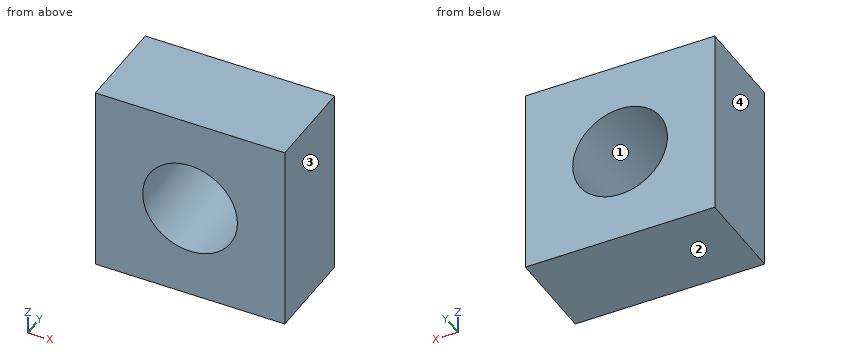
```python
from build123d import *

# Parameters (mm, degrees)
F0_W     = 20
F0_H     = 20
F1_DEPTH = 10
F2_R     = 5
F3_DEPTH = 10.001


with BuildPart() as f1:
    # F0 (on Front) → F1 (new body)
    with BuildSketch(Plane.XZ):
        Rectangle(F0_W, F0_H)
    extrude(amount=F1_DEPTH)

    # F2 (on face) → F3 (cut, through all)
    with BuildSketch(Plane.XZ.offset(10)):
        Circle(F2_R)
    extrude(amount=-F3_DEPTH, mode=Mode.SUBTRACT)


solid = f1.part
```
Geometry check sheet. Reference: the model listing, model coordinates, mm. Face numbers are marked on the shaded views. Give positions to 0.01 mm unless a question says otherwise; leave off trailing zeros. Loops run counter-clockwise (first coordinate to the right, second up) from the corner with the lowest first, then second, coordinate; pieces in that order, holes last. Notation, with made-up numbers: M -35,7.25 L 11,7.25 A34 cw 11,39.25 Z; hole C -7,29.5 d6. An arc over 180 degrees is marked long. Write item = value, one per line.
(1) Sectioned sample at B-B, the plane z = 0. Record the cut outline in (x, y), plus the area to 3 significant figures.
Answer below:
outline = M -10,-10 L -5,-10 L -5,0 L -10,0 Z; M 5,-10 L 10,-10 L 10,0 L 5,0 Z
area = 100 mm2
(2) Release check for a two-part mould opening along X. For the marked faces 1, 2, 3 and 4 record: released by +X, released by -X, zero draft, split by the parting line, or undercut.
Answer below:
face_1 = undercut
face_2 = zero draft
face_3 = released by +X
face_4 = released by -X
(3) Material ranges on line 1 (Z direction, x = 0, y = -2.75); line 2 (X direction, y = -9.25, z = 0.5); line 3 (X direction, y = -7, z = 0.75), recorded low to high. Write a range as [from, to].
Answer below:
line_1 = [-10, -5], [5, 10]
line_2 = [-10, -4.97], [4.97, 10]
line_3 = [-10, -4.94], [4.94, 10]
(4) Sectioned sample at C-C, the plane y = -2. Record the cut outline in (x, z).
Answer below:
outline = M -10,-10 L 10,-10 L 10,10 L -10,10 Z; hole C 0,0 d10
(5) Sectioned sample at A-A, the plane x = 0. Record the cut outline in (y, z), plus the area to 3 significant figures.
Answer below:
outline = M -10,-10 L 0,-10 L 0,-5 L -10,-5 Z; M -10,5 L 0,5 L 0,10 L -10,10 Z
area = 100 mm2
